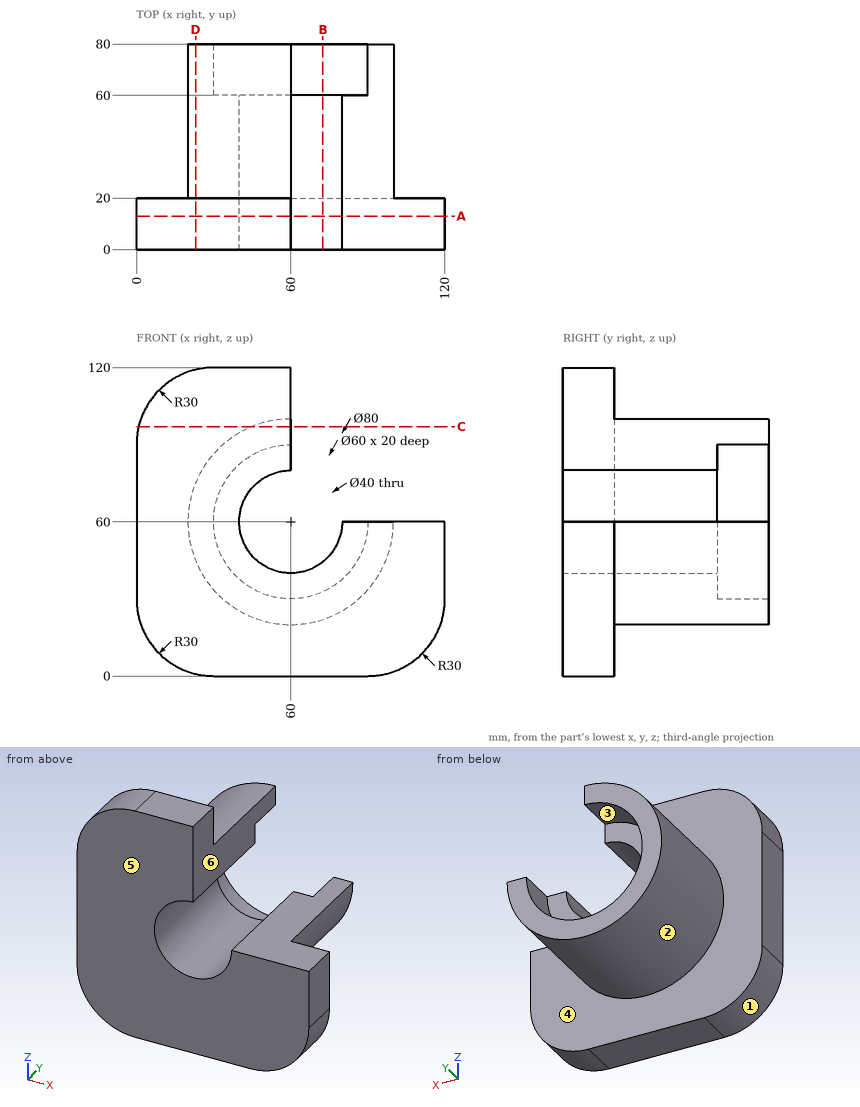
Study the drawing (mm; zero at the part's minimum x, y, z) and answer. A direction names the side the tool comes from. Give positions to 0.01 mm unless a question says otherwise; leave off trailing zeros. Write each loop counter-clockwise with the first axis right and the second up, starting at its lowest first coordinate (ties: lowest second). Pieces come first, ordered by that corner, then holes. Notation, with made-up numbers: (69, 33.25) - (124, 33.25) arc R8 cw to (124, 47.25) - close; hole circle Ø11 at (-14, 0.25). An arc over 180 degrees is marked (long way). Use a Markdown table: item, result.
1. Each of these flat-tipped pins is pushed along its axis until it touches: P1, Ø12, axis at x = 100.5, y = 32, coming from the +Z side; P2, Ø8, axis at x = 12.5, y = 13, coming from the -Z side; P3, Ø6, axis at x = 20.5, z = 105, coming from the -Y side; P4, Ø8, axis at x = 50, z = 104.5, coming from the +Y side. Where does it stop, or does it pass through?
Values follow:
| item | result |
|---|---|
| P1 | stops at z = 60 |
| P2 | stops at z = 3.21 |
| P3 | stops at y = 0 |
| P4 | stops at y = 20 |
2. For a pull along X with two mould halves and no side action, classify the marked faces 1, 2 and 3 as released by +X, released by -X, zero draft, split by the parting line, or undercut.
Values follow:
| item | result |
|---|---|
| face 1 | released by -X |
| face 2 | split by the parting line |
| face 3 | undercut |
3. A tool of negligible diameter and unlimited length cuts with its end or side. For the marked faces 4, 5 and 6, from which of +Z, -Z, +X, -X, +Y, -Y can it reach the whole face along a straight path? Write none if from no direction.
Values follow:
| item | result |
|---|---|
| face 4 | +Y |
| face 5 | +Z, -Z, +X, -X, -Y |
| face 6 | +Z, +X, +Y, -Y |
4. Section C-C on z = 97 is taken. Write down the section's boundary in (x, y), plus the area to 3 significant figures.
Values follow:
| item | result |
|---|---|
| outline | (0.83, 0) - (60, 0) - (60, 80) - (44.8, 80) - (44.8, 20) - (0.83, 20) - close |
| area | 2,100 mm² |
5. Section B-B on x = 72.5 is taken. Write down the section's boundary in (y, z), plus the area to 3 significant figures.
Values follow:
| item | result |
|---|---|
| outline | (0, 0) - (20, 0) - (20, 22) - (80, 22) - (80, 32.73) - (60, 32.73) - (60, 44.39) - (0, 44.39) - close |
| area | 2,000 mm² |
6. Section D-D on x = 23 is taken. Write down the section's boundary in (y, z), plus the area to 3 significant figures.
Values follow:
| item | result |
|---|---|
| outline | (0, 0.83) - (20, 0.83) - (20, 44.8) - (80, 44.8) - (80, 75.2) - (20, 75.2) - (20, 119.17) - (0, 119.17) - close |
| area | 4,190 mm² |
7. Find the intervals of material crossed by probe 1 along X at (y, z) = (62.5, 61.5); probe 2 along Y at (x, z) = (105.5, 24); probe 3 along Z at (x, y) = (53, 56.5) (3 decimals), in increasing order. Write a range as from..to.
Values follow:
| item | result |
|---|---|
| probe 1 | x = 20.03..30.04 |
| probe 2 | y = 0..20 |
| probe 3 | z = 20.617..41.265, 78.735..99.383 |
8. Section A-A on y = 13 is taken. Write down the section's boundary in (x, z).
Values follow:
| item | result |
|---|---|
| outline | (0, 30) arc R30 ccw to (30, 0) - (90, 0) arc R30 ccw to (120, 30) - (120, 60) - (80, 60) arc R20 cw (long way) to (60, 80) - (60, 120) - (30, 120) arc R30 ccw to (0, 90) - close |
